from build123d import *

# Parameters (mm, degrees)
SKETCH1_R           = 12.7
BOSS_EXTRUDE1_DEPTH = 17.5
SKETCH2_R           = 1.75
CUT_EXTRUDE1_DEPTH  = 10
CIRPATTERN1_COUNT   = 4
CIRPATTERN7_COUNT   = 21
SKETCH5_R           = 19.84375
CUT_EXTRUDE5_DEPTH  = 5.95
SKETCH9_R           = 2
CUT_EXTRUDE11_DEPTH = 26
CIRPATTERN9_COUNT   = 4
SKETCH10_R          = 1.5
CUT_EXTRUDE12_DEPTH = 26
SKETCH11_R          = 1.5
CUT_EXTRUDE13_DEPTH = 30


with BuildPart() as part:
    # Sketch1 → Boss-Extrude1 (new body)
    with BuildSketch(Plane.XY):
        with BuildLine():
            Line((-1.845299462, 24.299103121), (-3, 22.299103121))
            ThreePointArc((-3, 22.299103121), (0, -22.5), (3, 22.299103121))
            Line((3, 22.299103121), (1.845299462, 24.299103121))
            Line((1.845299462, 24.299103121), (-1.845299462, 24.299103121))
        make_face()
        Circle(SKETCH1_R, mode=Mode.SUBTRACT)
    boss_extrude1 = extrude(amount=BOSS_EXTRUDE1_DEPTH)

    # Sketch2 → Cut-Extrude1 (cut)
    with BuildSketch(Plane.XY.offset(17.5)):
        with Locations((-11.6, 11.6)):
            Circle(SKETCH2_R)
    cut_extrude1 = extrude(amount=-CUT_EXTRUDE1_DEPTH, mode=Mode.SUBTRACT)

    # CirPattern1: Cut-Extrude1 ×4 about axis
    cirpattern1_axis = Axis((0, 0, 0), (0, 0, 1))
    for i in range(1, CIRPATTERN1_COUNT):
        add(cut_extrude1.rotate(cirpattern1_axis, i * 360 / CIRPATTERN1_COUNT), mode=Mode.SUBTRACT)

    # CirPattern7: Boss-Extrude1 ×21 about axis
    cirpattern7_axis = Axis((0, 0, 0), (0, 0, 1))
    for i in range(1, CIRPATTERN7_COUNT):
        add(boss_extrude1.rotate(cirpattern7_axis, i * 360 / CIRPATTERN7_COUNT))

    # Sketch5 → Cut-Extrude5 (cut)
    with BuildSketch(Plane(origin=(0, 0, 0), x_dir=(-1, 0, 0), z_dir=(0, 0, -1))):
        Circle(SKETCH5_R)
    extrude(amount=-CUT_EXTRUDE5_DEPTH, mode=Mode.SUBTRACT)

    # Sketch9 → Cut-Extrude11 (cut)
    with BuildSketch(Plane(origin=(0, 0, 5.95), x_dir=(-1, 0, 0), z_dir=(0, 0, -1))):
        with Locations((0, 16)):
            Circle(SKETCH9_R)
    cut_extrude11 = extrude(amount=-CUT_EXTRUDE11_DEPTH, mode=Mode.SUBTRACT)

    # CirPattern9: Cut-Extrude11 ×4 about axis
    cirpattern9_axis = Axis((0, 0, 0), (0, 0, 1))
    for i in range(1, CIRPATTERN9_COUNT):
        add(cut_extrude11.rotate(cirpattern9_axis, i * 360 / CIRPATTERN9_COUNT), mode=Mode.SUBTRACT)

    # Sketch10 → Cut-Extrude12 (cut)
    with BuildSketch(Plane(origin=(13.688172181, 20.07686118, 0), x_dir=(0.8262387743160019, -0.5633200580636119, 0), z_dir=(0.5633200580636117, 0.8262387743160018, 0))):
        with Locations(Location((-0.048095596, -8.999871489, 0), (0, 0, 180))):
            Circle(SKETCH10_R)
    extrude(amount=-CUT_EXTRUDE12_DEPTH, mode=Mode.SUBTRACT)

    # Sketch11 → Cut-Extrude13 (cut)
    with BuildSketch(Plane(origin=(0, 24.299103121, 0), x_dir=(1, 0, 0), z_dir=(0, 1, 0))):
        with Locations(Location((0, -9.826057875, 0), (0, 0, 270))):
            Circle(SKETCH11_R)
    extrude(amount=-CUT_EXTRUDE13_DEPTH, mode=Mode.SUBTRACT)


solid = part.part
Here's how the part is built. I have some questions about the finished solid (model axes, mm). A direction names the side the tool comes from. Coordinates: 2 decimals unless noted, no trailing zeros.
Item 1: For P1, Ø2, axis at x = -4.5, y = 9, coming from the -Z side; P2, Ø1.5, axis at x = -3.5, z = 3.5, coming from the +Y side; P3, Ø1.2, axis at x = 19.5, z = 10, coming from the -Y side; P4, Ø2.5, axis at x = 0, z = 9.83, coming from the +Y side, each with a flat end and sliding along its axis, tell me the tip position at first contact or that it passes through.
Result sheet:
P1: passes through
P2: stops at y = 22.73
P3: stops at y = -13.75
P4: stops at y = -12.64
Item 2: For faces 4 (the face through (23.266, -2.834, 8.628)), 5 (the face through (-14.087, -18.732, 8.628)), 6 (the face through (-23.428, -0.666, 8.628)), which set-ups out of +Z, -Z, +X, -X, +Y, -Y let a thin tool reach every point of the face, with its end or its side?
Result sheet:
face 4: +Z, -Z, +X
face 5: +Z, -Z, -Y
face 6: +Z, -Z, -X
Item 3: I need wall thicknesses on line 1 (X direction, y = 0, z = 12.25); line 2 (Z direction, x = 0, y = 19); line 3 (Y direction, x = 0, z = 1.6). Which ranges of each line are inside material? Lowest first, please.
Result sheet:
line 1: x = -24.37 to -18, -14 to -12.7, 12.7 to 14, 18 to 24.37
line 2: z = 5.95 to 8.33, 11.33 to 17.5
line 3: y = -22.5 to -19.84, 19.84 to 24.3
Item 4: If we mould it in two halves opening along Y, with no side actions, what happens to faces 1 (the face through (19.72, 12.62, 8.63)), 2 (the face through (7.19, 23.21, 8.63)), 3 (the face through (-12.293, -19.924, 8.628))? For each: +Y half, -Y half, draft (parallel to the pull), parting line (faces both ways), or undercut.
Result sheet:
face 1: undercut
face 2: +Y half
face 3: -Y half
Item 5: If we section it at A-A on z = 15.5: State how many separate pieces and enclosed holes the cut face has, plus the area to 3 significant figures.
Result sheet:
separate pieces: 1
enclosed holes: 5
area: 1,220 mm2
